Could you check a few things on this model? Use its own coordinates, in mm. A direction names the side the tool comes from. Give positions to 0.01 mm unless a question says otherwise; leave off trailing zeros. Write each loop counter-clockwise with the first axis right and the second up, starting at its lowest first coordinate (ties: lowest second). Pieces come first, ordered by that corner, then holes. Notation, with made-up numbers: (26, 29) - (47, 29) arc R24 cw to (47, 66) - close; hole circle Ø11 at (48.5, -24.75). An arc over 180 degrees is marked (long way). Answer as CSV lines item,"result". Start each with the question number.
Q1. We'd pull the mould along X, two halves only. Please class faces 1 (the face through (0, 35, 5)), 2 (the face through (-0.1, 0, 3.4)), 3 (the face through (5.021, 31.198, 16.085)): pulls with the +X half, pulls with the -X half, needs draft (parallel to the pull), parting line crosses it, or undercut.
Q2. Imagine slicing it at A-A on z = 18.5. List the corners of the cut face in (x, y) for me, and give its area (3 significant figures).
Q3. Imagine slicing it at C-C on x = -13.5. List the corners of the cut face in (y, z) for me, and give its area (3 significant figures).
Q4. Imagine slicing it at B-B on y = 16. List the corners of the cut face in (x, z) for me.
Q5. Will these pins go through, and if not, where does the flat tip stop? pin 1 Ø3 at (x, y) = (5.5, 18.5) entering from +Z; pin 2 Ø2.5 at (x, y) = (9, 16) entering from +Z; pin 3 Ø2 at (x, y) = (0.5, 31.5) entering from +Z; pin 4 Ø6 at (y, z) = (33, 8.5) entering from +X.
Q6. On a 3-axis mill with a long thin cutter (end or side, diameter ignored), from which of +Z, -Z, +X, -X, +Y, -Y can I reach the whole of each face in a straight line? I mean faces 4 (the face through (-5.021, 31.198, 16.085)), 5 (the face through (13.23, -24.72, 9.86)), 6 (the face through (-0.423, 28.423, 13.222)), 7 (the face through (6.5, 31, 7)), 8 (the face through (9, 10, 9)). Say none if no direction works.
Q7. If I drill on line 1 along Y through (x, z) = (-7.5, 8); line 2 along Z through (x, y) = (0, -26.3); line 3 along Z through (x, y) = (0, 29.25), over which ranges is the centre line in solid material (lowest first)?
Q8. Imagine slicing it at D-D on z = 12.5. State how many separate pieces and enclosed holes the cut face has, and give its area (3 significant figures).
```python
from build123d import *

# Parameters (mm, degrees)
F0_W           = 35
F0_H           = 55
F0_R           = 1.25
F1_DEPTH       = 20
F2_DEPTH       = 3
F3_R           = 1
F4_W           = 3
F4_H           = 20
F5_DEPTH       = 15
F7_DEPTH       = 5.5
F8_R           = 2.1
F9_DEPTH       = 25
F9_DEPTH_BACK  = 25
F10_R          = 5.25
F11_DEPTH      = 25
F11_DEPTH_BACK = 30
F13_START      = -23
F12_W          = 13
F12_H          = 17.6061931998
F12_R          = 3.25
F13_DEPTH      = 12
F14_DEPTH      = 25
F14_DEPTH_BACK = 25
F15_SIZE       = 3
F16_R          = 1


with BuildPart() as f1:
    # F0 (on Top) → F1 (new body)
    with BuildSketch(Plane.XY):
        Rectangle(F0_W, F0_H)
        with Locations((-13.5, -23.5)):
            Circle(F0_R, mode=Mode.SUBTRACT)
        with Locations((13.5, -23.5)):
            Circle(F0_R, mode=Mode.SUBTRACT)
        with Locations((-13.5, 23.5)):
            Circle(F0_R, mode=Mode.SUBTRACT)
        with BuildLine():
            ThreePointArc((15, -19), (10.7573593129, -20.7573593129), (9, -25))
            Line((9, -25), (-9, -25))
            ThreePointArc((-9, -25), (-10.7573593129, -20.7573593129), (-15, -19))
            Line((-15, -19), (-15, 19))
            ThreePointArc((-15, 19), (-10.7573593129, 20.7573593129), (-9, 25))
            Line((-9, 25), (9, 25))
            ThreePointArc((9, 25), (10.7573593129, 20.7573593129), (15, 19))
            Line((15, 19), (15, -19))
        make_face(mode=Mode.SUBTRACT)
        with Locations((13.5, 23.5)):
            Circle(F0_R, mode=Mode.SUBTRACT)
    extrude(amount=F1_DEPTH)

    # F0 (on Top) → F2 (join)
    with BuildSketch(Plane.XY):
        with BuildLine():
            Line((-9, -25), (9, -25))
            ThreePointArc((9, -25), (10.7573593129, -20.7573593129), (15, -19))
            Line((15, -19), (15, 19))
            ThreePointArc((15, 19), (10.7573593129, 20.7573593129), (9, 25))
            Line((9, 25), (-9, 25))
            ThreePointArc((-9, 25), (-10.7573593129, 20.7573593129), (-15, 19))
            Line((-15, 19), (-15, -19))
            ThreePointArc((-15, -19), (-10.7573593129, -20.7573593129), (-9, -25))
        make_face()
    extrude(amount=F2_DEPTH)

    # F3
    f3_edges = [f1.edges().sort_by_distance(p)[0] for p in [
        (17.5, 27.5, 10),
        (-17.5, 27.5, 10),
        (17.5, -27.5, 10),
        (-17.5, -27.5, 10),
    ]]
    fillet(f3_edges, radius=F3_R)

    # F4 (on Top) → F5 (join)
    with BuildSketch(Plane.XY):
        with Locations((-8.75, 0)):
            Rectangle(F4_W, F4_H)
        with Locations((8.75, 0)):
            Rectangle(F4_W, F4_H)
    extrude(amount=F5_DEPTH)

    # F6 (on Top) → F7 (join)
    with BuildSketch(Plane.XY):
        Polygon((-9, 0), (0, 0), (9, 0), (9, 4), (-9, 4), align=None)
    extrude(amount=F7_DEPTH)

    # F8 (on Top) → F9 (cut, two sides)
    with BuildSketch(Plane.XY) as f9_sk:
        with Locations((-9, 16)):
            Circle(F8_R)
        with Locations((9, 16)):
            Circle(F8_R)
    extrude(amount=-F9_DEPTH, mode=Mode.SUBTRACT)
    extrude(f9_sk.sketch, amount=F9_DEPTH_BACK, mode=Mode.SUBTRACT)

    # F10 (on Front) → F11 (cut, two sides)
    with BuildSketch(Plane.XZ) as f11_sk:
        with Locations((0, 9)):
            Circle(F10_R)
    extrude(amount=-F11_DEPTH, mode=Mode.SUBTRACT)
    extrude(f11_sk.sketch, amount=F11_DEPTH_BACK, mode=Mode.SUBTRACT)

    # F12 (on Front) → F13 (join)
    with BuildSketch(Plane.XZ.offset(F13_START)):
        with Locations((0, 8.8030965999)):
            Rectangle(F12_W, F12_H)
        with Locations((0, 10)):
            Circle(F12_R, mode=Mode.SUBTRACT)
    extrude(amount=-F13_DEPTH)

    # F14 (cut, two sides): a face of the model
    f14_faces = [f1.faces().sort_by_distance(p)[0] for p in [
        (0, 27.5, 10),
    ]]
    extrude(f14_faces, amount=-F14_DEPTH, mode=Mode.SUBTRACT)
    extrude(f14_faces, amount=F14_DEPTH_BACK, mode=Mode.SUBTRACT)

    # F15
    f15_edges = [f1.edges().sort_by_distance(p)[0] for p in [
        (6.5, 31.25, 17.606193),
        (-6.5, 31.25, 17.606193),
    ]]
    chamfer(f15_edges, length=F15_SIZE)

    # F16
    f16_edges = [f1.edges().sort_by_distance(p)[0] for p in [
        (-3.25, 35, 10),
        (-5.25, -25, 9),
        (-7.25, 0, 15),
        (7.25, 0, 15),
    ]]
    fillet(f16_edges, radius=F16_R)


solid = f1.part
```
Conclusion:
1,face 1,"needs draft"
1,face 2,"undercut"
1,face 3,"pulls with the +X half"
2,outline,"(-17.5, -26.5) arc R1 ccw to (-16.5, -27.5) - (16.5, -27.5) arc R1 ccw to (17.5, -26.5) - (17.5, 26.5) arc R1 ccw to (16.5, 27.5) - (-16.5, 27.5) arc R1 ccw to (-17.5, 26.5) - close; hole (-15, -19) arc R6 cw to (-9, -25) - (9, -25) arc R6 cw to (15, -19) - (15, 19) arc R6 cw to (9, 25) - (-9, 25) arc R6 cw to (-15, 19) - close; hole circle Ø2.5 at (-13.5, -23.5); hole circle Ø2.5 at (-13.5, 23.5); hole circle Ø2.5 at (13.5, -23.5); hole circle Ø2.5 at (13.5, 23.5)"
2,area,"518 mm^2"
3,outline,"(-27.5, 0) - (-24.75, 0) - (-24.75, 20) - (-27.5, 20) - close; (-22.25, 0) - (22.25, 0) - (22.25, 20) - (19.19, 20) - (19.19, 3) - (-19.19, 3) - (-19.19, 20) - (-22.25, 20) - close; (24.75, 0) - (27.5, 0) - (27.5, 20) - (24.75, 20) - close"
3,area,"348 mm^2"
4,outline,"(-17.5, 0) - (-11.1, 0) - (-11.1, 3) - (-15, 3) - (-15, 20) - (-17.5, 20) - close; (-6.9, 0) - (6.9, 0) - (6.9, 3) - (-6.9, 3) - close; (11.1, 0) - (17.5, 0) - (17.5, 20) - (15, 20) - (15, 3) - (11.1, 3) - close"
5,pin 1,"z = 3"
5,pin 2,"through"
5,pin 3,"z = 17.61"
5,pin 4,"x = 6.5"
6,face 4,"+Z, -X, +Y"
6,face 5,"+Z, -Z"
6,face 6,"+Y, -Y"
6,face 7,"+Z, -Z, +X, +Y"
6,face 8,"+Z"
7,line 1,"-27.5 to -25, -10 to 10, 25 to 27.5"
7,line 2,"0 to 3.75, 14.25 to 20"
7,line 3,"0 to 6.75, 13.25 to 17.61"
8,separate pieces,"4"
8,enclosed holes,"4"
8,area,"691 mm^2"
